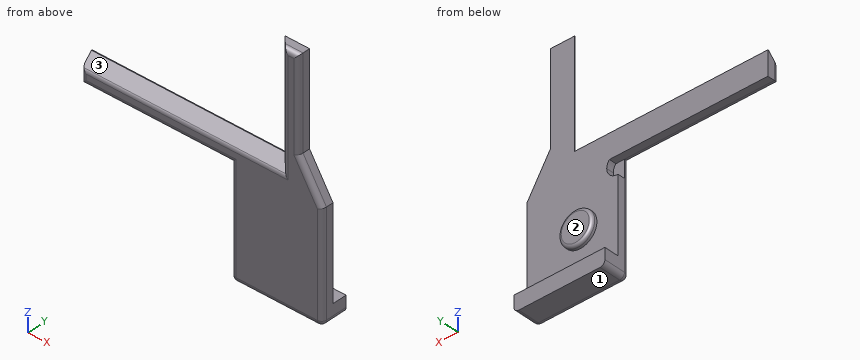
```python
from build123d import *

# Parameters (mm, degrees)
F0_W          = 37.648660762
F0_H          = 6.6216221157
F1_DEPTH      = 6
F1_DEPTH_BACK = 5
F0_R          = 7
F2_DEPTH      = 5
F3_DEPTH      = 2.2
F4_SIZE       = 4.7
F5_R          = 1.2
F6_R          = 2
F8_DEPTH      = 2
F8_DEPTH_BACK = 3


with BuildPart() as f1:
    # F0 (on Front) → F1 (new body, two sides)
    with BuildSketch(Plane.XZ) as f1_sk:
        with Locations((37.9482610798, -64.9883002128)):
            Rectangle(F0_W, F0_H)
    extrude(amount=-F1_DEPTH)
    extrude(f1_sk.sketch, amount=F1_DEPTH_BACK)

    # F0 (on Front) → F2 (join)
    with BuildSketch(Plane.XZ):
        Polygon((19.1239306988, -23.4612585763), (19.1239306988, -61.677489155), (56.7725914607, -61.677489155), (56.7725914607, -23.4612585763), (47.0698534062, -23.4612585763), (37.0698534062, -23.4612585763), align=None)
        with Locations((34.8266364816, -44.477489155)):
            Circle(F0_R, mode=Mode.SUBTRACT)
        Polygon((-42.9301465938, -23.4612585763), (19.1239306988, -23.4612585763), (37.0698534062, -23.4612585763), (37.0698534062, -13.4612585763), (-42.9301465938, -13.4612585763), align=None)
        Polygon((37.0698534062, -13.4612585763), (37.0698534062, -23.4612585763), (47.0698534062, -23.4612585763), (47.0698534062, -7.6851719059), (47.0698534062, 30.268489238), (37.0698534062, 30.268489238), align=None)
        with Locations((34.8266364816, -44.477489155)):
            Circle(F0_R)
        Polygon((47.0698534062, -23.4612585763), (56.7725914607, -23.4612585763), (47.0698534062, -7.6851719059), align=None)
    extrude(amount=F2_DEPTH)

    # F0 (on Front) → F3 (join)
    with BuildSketch(Plane.XZ):
        with Locations((34.8266364816, -44.477489155)):
            Circle(F0_R)
    extrude(amount=-F3_DEPTH)

    # F4
    f4_edges = [f1.edges().sort_by_distance(p)[0] for p in [
        (-2.930147, -5, -13.461259),
        (37.069853, -5, 8.403615),
    ]]
    chamfer(f4_edges, length=F4_SIZE)

    # F5
    f5_edges = [f1.edges().sort_by_distance(p)[0] for p in [
        (27.826636, 2.2, -44.477489),
    ]]
    fillet(f5_edges, radius=F5_R)

    # F6
    f6_edges = [f1.edges().sort_by_distance(p)[0] for p in [
        (51.921222, -5, -15.573215),
        (47.069853, -5, 11.291659),
        (56.772591, -5, -45.880185),
        (37.948261, -5, -68.299111),
        (44.419853, -5, 30.268489),
        (41.769853, -5, 6.053615),
        (-0.580147, -5, -18.161259),
        (-42.930147, -5, -20.811259),
        (-11.903108, -5, -23.461259),
        (19.123931, -5, -45.880185),
        (19.123931, 0.5, -68.299111),
        (56.772591, 0.5, -68.299111),
    ]]
    fillet(f6_edges, radius=F6_R)

    # F7 (on face) → F8 (cut, two sides)
    with BuildSketch(Plane.XZ) as f8_sk:
        with BuildLine():
            ThreePointArc((19.1239306988, -30.7265526876), (22.3891362533, -29.5527672873), (23.7676569653, -26.3685844839))
            ThreePointArc((23.7676569653, -26.3685844839), (23.4811232341, -24.8128381171), (22.6591250093, -23.4612585763))
            Line((22.6591250093, -23.4612585763), (19.1239306988, -23.4612585763))
            Line((19.1239306988, -23.4612585763), (19.1239306988, -30.7265526876))
        make_face()
    extrude(amount=-F8_DEPTH, mode=Mode.SUBTRACT)
    extrude(f8_sk.sketch, amount=F8_DEPTH_BACK, mode=Mode.SUBTRACT)


solid = f1.part
```
The listing builds one solid part. Answer for the finished solid, in the listing's coordinates (mm). Face numbers are marked on the shaded views. A direction names the side the tool comes from. Give positions to 0.01 mm unless a question says otherwise; leave off trailing zeros. Write each loop counter-clockwise with the first axis right and the second up, starting at its lowest first coordinate (ties: lowest second). Pieces come first, ordered by that corner, then holes. Notation, with made-up numbers: M 24.25,34 L 77.25,34 A24 cw 77.25,58 Z; hole C 23,-16.5 d7. An arc over 180 degrees is marked long. Write each question's results on one line, items separated by ' | '.
Q1. Flat-ended cylindrical pins translate along their axes: P1, Ø4.5, axis at y = 1.5, z = -46, coming from the -X side; P2, Ø4, axis at y = -1, z = 19.5, coming from the -X side; P3, Ø0.9, axis at x = -14.5, y = -1.5, coming from the -Z side; P4, Ø6.5, axis at x = 41.5, y = 2, coming from the +Z side. Find the tip coordinate at first contact, or state that the pin passes through.
Output values:
P1: x = 19.12 | P2: x = 37.07 | P3: z = -23.46 | P4: z = 30.27
Q2. Section A-A, the plane z = 4.5 is taken. Write down the section's boundary in (x, y).
Output values:
outline: M 37.07,-0.3 L 41.18,-4.41 A2 ccw 42.6,-5 L 45.07,-5 A2 ccw 47.07,-3 L 47.07,0 L 37.07,0 Z
Q3. A tool of negligible diameter and unlimited length cuts with its end or side. For the marked faces 1, 2 and 3, from which of +Z, -Z, +X, -X, +Y, -Y can it reach the whole face along a straight path? Write none if from no direction.
Output values:
face 1: -Z, +X, -X, +Y, -Y | face 2: +Z, +X, -X, +Y | face 3: +Z, -X, -Y
Q4. Consider L1, parallel to Y at x = 36, z = -39; L2, parallel to Z at x = 24.5, y = 0.75; L3, parallel to X at y = -2.25, z = -63. Determine where each line is inside the solid, lowest interval first. Write a range as from..to.
Output values:
L1: -5..2.2 | L2: -68.3..-61.68 | L3: 19.12..56.77
Q5. Section B-B, the plane x = -27 is taken. Write down the section's boundary in (y, z), then the cut area to 3 significant figures.
Output values:
outline: M -5,-21.46 A2 ccw -3,-23.46 L 0,-23.46 L 0,-13.46 L -0.3,-13.46 L -4.41,-17.58 A2 ccw -5,-18.99 Z | area: 38.0 mm2
Q6. Section C-C, the plane y = 4 is taken. Write down the section's boundary in (x, z), then the cut area to 3 significant figures.
Output values:
outline: M 19.12,-66.3 A2 ccw 21.12,-68.3 L 54.77,-68.3 A2 ccw 56.77,-66.3 L 56.77,-61.68 L 19.12,-61.68 Z | area: 248 mm2
